CAD build for the part. Positions are in the model's coordinates, mm. Give positions to 0.01 mm unless a question says otherwise; leave off trailing zeros. Write each loop counter-clockwise with the first axis right and the second up, starting at its lowest first coordinate (ties: lowest second). Pieces come first, ordered by that corner, then holes. Notation, with made-up numbers: (53, -0.5) - (94, -0.5) arc R26 cw to (94, 38.5) - close; hole circle Ø10 at (58.25, 34.5). An arc over 180 degrees is marked (long way). Answer as a JSON object with one key per item and string values.
from build123d import *

# Parameters (mm, degrees)
SKETCH_2_R      = 5
SKETCH_2_R_2    = 2.5
EXTRUDE_1_DEPTH = 5


with BuildPart() as part:
    # 草图2 → 凸台-拉伸1 (new body)
    # profile 1 of 3: a face of its own
    with BuildSketch(Plane(origin=(0, 0, 0), x_dir=(1, 0, 0), z_dir=(0, 1, 0))):
        with BuildLine():
            ThreePointArc((5, 0), (3.535533906, -3.535533906), (0, -5))
            Line((0, -5), (207.06, -5))
            ThreePointArc((207.06, -5), (202.06, 0), (207.06, 5))
            Line((207.06, 5), (0, 5))
            ThreePointArc((0, 5), (3.535533906, 3.535533906), (5, 0))
        make_face()
    # profile 2 of 3: a face of its own
    with BuildSketch(Plane(origin=(0, 0, 0), x_dir=(1, 0, 0), z_dir=(0, 1, 0))):
        Circle(SKETCH_2_R)
        with Locations(Location((0, 0, 0), (0, 0, 270))):
            Circle(SKETCH_2_R_2, mode=Mode.SUBTRACT)
    # profile 3 of 3: a face of its own
    with BuildSketch(Plane(origin=(0, 0, 0), x_dir=(1, 0, 0), z_dir=(0, 1, 0))):
        with Locations((207.06, 0)):
            Circle(SKETCH_2_R)
        with Locations(Location((207.06, 0, 0), (0, 0, 270))):
            Circle(SKETCH_2_R_2, mode=Mode.SUBTRACT)
    extrude(amount=EXTRUDE_1_DEPTH)


solid = part.part
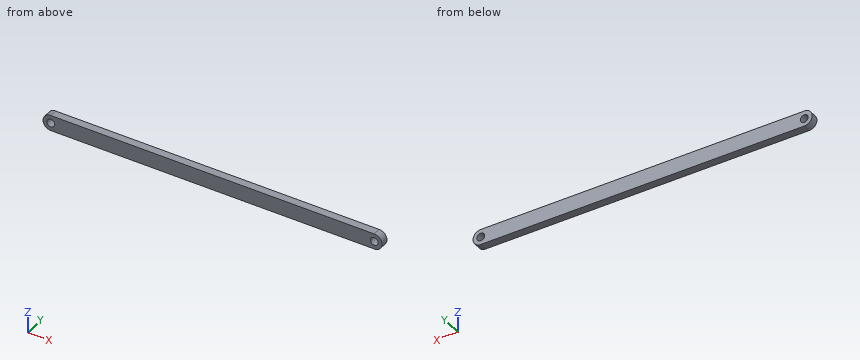
Item 1: Cut at A-A (z = 0). Give the cut face in (x, y).
Entries:
{"outline": "(-5, 0) - (-2.5, 0) - (-2.5, 5) - (-5, 5) - close; (2.5, 0) - (204.56, 0) - (204.56, 5) - (2.5, 5) - close; (209.56, 0) - (212.06, 0) - (212.06, 5) - (209.56, 5) - close"}
Item 2: Cut at B-B (y = 1.8). Give the cut face in (x, z).
Entries:
{"outline": "(0, -5) - (207.06, -5) arc R5 ccw to (207.06, 5) - (0, 5) arc R5 ccw to start; hole circle Ø5 at (0, 0); hole circle Ø5 at (207.06, 0)"}
Item 3: Flat gauge pins, fed straight in: P1, Ø1.5, axis at y = 1.5, z = -1, coming from the -X side; P2, Ø4, axis at x = 0, z = 0, coming from the -Y side; P3, Ø1, axis at y = 2.5, z = 1.5, coming from the +X side. Where does each tip first touch, or does it go through?
Entries:
{"P1": "x = -4.99", "P2": "through", "P3": "x = 211.96"}
Item 4: Probe line 1 (X direction, y = 2.8, z = 0); line 2 (X direction, y = 1.75, z = -1); line 3 (Z direction, x = 207.06, y = 1.9). List the from-to ranges inside material, lowest first. Write a range as from..to.
Entries:
{"line 1": "-5..-2.5, 2.5..204.56, 209.56..212.06", "line 2": "-4.9..-2.29, 2.29..204.77, 209.35..211.96", "line 3": "-5..-2.5, 2.5..5"}
